For this review, use the dimensioned drawing (mm, ordinates from the lowest corner) and the shaded views. Round coordinates to 2 decimals unless told otherwise and drop trailing zeros. Order: outer loops, then holes, each group sorted by start corner. A loop starts at its lowest first (then second) coordinate and runs counter-clockwise, first axis right, second up. Notation, with made-up numbers: M 81,29 L 133,29 A10 cw 133,41 Z; hole C 31,24 d8. An arc over 180 degrees is marked long. Put each result on its own line as item: value.
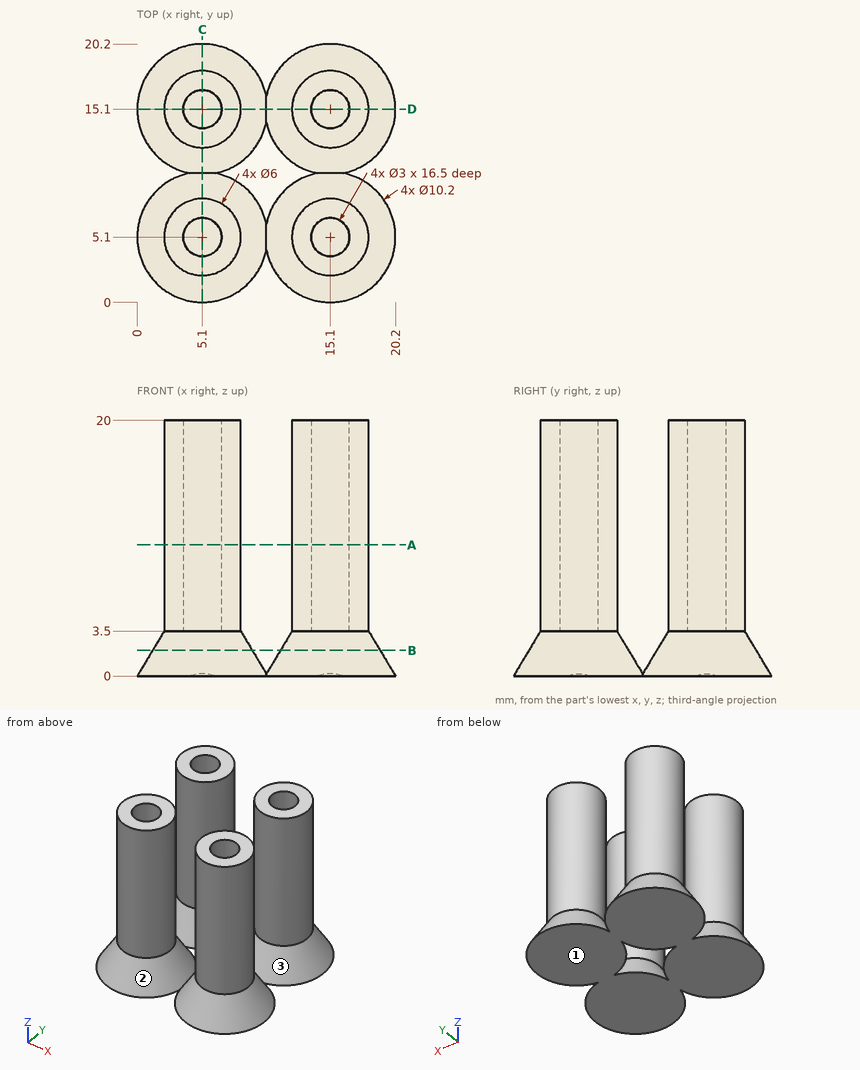
(1) Add section B-B on z = 2. Give the boundary of the cut face in (x, y).
A:
outline: C 5.1,5.1 d7.8; C 5.1,15.1 d7.8; C 15.1,5.1 d7.8; C 15.1,15.1 d7.8
(2) To check wall thickness, follow L1, parallel to Y at x = 15.1, z = 15.5; L2, parallel to Y at x = 5.5, z = 9.75. State the ranges of each line that lie inside material, in increasing order.
A:
L1: y = 2.1 to 3.6, 6.6 to 8.1, 12.1 to 13.6, 16.6 to 18.1
L2: y = 2.13 to 3.65, 6.55 to 8.07, 12.13 to 13.65, 16.55 to 18.07
(3) Add section C-C on x = 5.1. Give the boundary of the cut face in (y, z).
A:
outline: M 0,0 L 20.2,0 L 18.1,3.5 L 18.1,20 L 16.6,20 L 16.6,3.5 L 13.6,3.5 L 13.6,20 L 12.1,20 L 12.1,3.5 L 10.1,0.17 L 8.1,3.5 L 8.1,20 L 6.6,20 L 6.6,3.5 L 3.6,3.5 L 3.6,20 L 2.1,20 L 2.1,3.5 Z
(4) Add section A-A on z = 10.25. Give the boundary of the cut face in (x, y), then the cut area to 3 significant figures.
A:
outline: C 5.1,5.1 d6; C 5.1,15.1 d6; C 15.1,5.1 d6; C 15.1,15.1 d6; hole C 5.1,5.1 d3; hole C 5.1,15.1 d3; hole C 15.1,5.1 d3; hole C 15.1,15.1 d3
area: 84.8 mm2
(5) Draft analysis for pull direction Y (two halves, no side actions). For the marked faces 1, 2 and 3, state which applies: released by +Y, released by -Y, zero draft, split by the parting line, or undercut.
A:
face 1: zero draft
face 2: undercut
face 3: undercut
(6) Insertion check: pin 1 Ø4 at (y, z) = (14, 12.5) entering from +X; pin 2 Ø1.5 at (x, y) = (5.5, 15) entering from +Z; pin 3 Ø1.5 at (x, y) = (12, 9.5) entering from +Z. Each pin has a flat end and moves straight along its axis. Give the tip position at first contact, or say it passes through.
A:
pin 1: stops at x = 18.1
pin 2: stops at z = 3.5
pin 3: stops at z = 0.78
